CAD build for the part. Positions are in the model's coordinates, mm. A direction names the side the tool comes from. Coordinates: 2 decimals unless noted, no trailing zeros. Loops run counter-clockwise (first coordinate to the right, second up) from the corner with the lowest first, then second, coordinate; pieces in that order, holes last. Notation, with made-up numbers: (71, -8.5) -> (98, -8.5) arc R14 cw to (98, 14.5) -> close; hole circle Ø9 at (-27, -40). An arc over 180 degrees is marked (long way). Write item = value, one per line. Start each with the question number.
(1) Drill centre lines: line 1 (Y direction, x = -2.5, z = 6.5); line 2 (X direction, y = 4.5, z = 7.5); line 3 (X direction, y = 8, z = 2.25). Where is each one in solid material? Low to high. Write a range as from..to.
(2) Tool access for faces 1 (the face through (-8.264, 19.366, 2.075)), 2 (the face through (6.115, 17.736, -1.524)), 3 (the face through (1.237, 24.566, 6.484)): list every direction of +Z, -Z, +X, -X, +Y, -Y with a clear straight run to the whole face (end or side of a thin tool).
(3) Band-saw the part on A-A (y = 3.5). Write the cut outline in (x, z).
(4) Band-saw the part on D-D (y = 6.5). Write the cut outline in (x, z), and give its area (3 significant figures).
(5) Pull direction Z, two halves, no side cores. Call faces 4 (the face through (3, 13, -3.839)), 5 (the face through (6.115, 7.986, -1.524)), 6 (the face through (1.59, 13.31, -0.61)): +Z half, -Z half, draft (parallel to the pull), parting line (faces both ways), or undercut.
(6) Band-saw the part on C-C (z = 2). Count the separate pieces of the cut face and the enclosed holes in it, and give its area (3 significant figures).
(7) Band-saw the part on B-B (x = -3.5). Write the cut outline in (y, z), and give its area (3 significant figures).
(8) Flat gauge pin, fed straight in: P1, Ø2.5, axis at x = 9.94, y = 3.5, coming from the -Z side. Where does the tip first touch, or does it go through?
```python
from build123d import *

# Parameters (mm, degrees)
EXTRUDE_1_DEPTH        = 7
SKETCH_2_R             = 5
EXTRUDE_2_DEPTH        = 15
EXTRUDE_3_DEPTH        = 1.25
PATTERN_LINEAR_1_COUNT = 4
PATTERN_LINEAR_1_PITCH = 3.25
EXTRUDE_5_DEPTH        = 5
SKETCH_8_R             = 1.6
CUT_EXTRUDE_2_DEPTH    = 33.583240961
SKETCH_9_R             = 1.5
CUT_EXTRUDE_3_DEPTH    = 5
SKETCH_10_R            = 3
CUT_EXTRUDE_4_DEPTH    = 32.373048931


with BuildPart() as part:
    # 草图1 → 凸台-拉伸1 (new body)
    with BuildSketch(Plane(origin=(0, 0, 0), x_dir=(1, 0, 0), z_dir=(0, 1, 0))):
        with BuildLine():
            Line((-7.264367816, 3.83908046), (12.735632184, 3.83908046))
            ThreePointArc((12.735632184, 3.83908046), (13.735632184, -2.16091954), (12.735632184, -8.16091954))
            Line((12.735632184, -8.16091954), (-7.264367816, -8.16091954))
            ThreePointArc((-7.264367816, -8.16091954), (-8.264367816, -2.16091954), (-7.264367816, 3.83908046))
        make_face()
    extrude(amount=EXTRUDE_1_DEPTH)

    # 草图2 → 凸台-拉伸2 (add)
    with BuildSketch(Plane(origin=(0, 7, 0), x_dir=(1, 0, 0), z_dir=(0, 1, 0))):
        with Locations(Location((2.735632184, -2.16091954, 0), (0, 0, 270))):
            Circle(SKETCH_2_R)
    extrude(amount=EXTRUDE_2_DEPTH)

    # 草图4 → 凸台-拉伸3 (add)
    with BuildSketch(Plane(origin=(0, 9, 0), x_dir=(1, 0, 0), z_dir=(0, 1, 0))):
        with BuildLine():
            Line((-7.264367816, -8.16091954), (12.735632184, -8.16091954))
            ThreePointArc((12.735632184, -8.16091954), (13.735632184, -2.16091954), (12.735632184, 3.83908046))
            Line((12.735632184, 3.83908046), (-7.264367816, 3.83908046))
            ThreePointArc((-7.264367816, 3.83908046), (-8.264367816, -2.16091954), (-7.264367816, -8.16091954))
        make_face()
    extrude_3 = extrude(amount=EXTRUDE_3_DEPTH)

    # 阵列(线性)1: 凸台-拉伸3 ×4
    with Locations(*[(0, i * PATTERN_LINEAR_1_PITCH, 0) for i in range(1, PATTERN_LINEAR_1_COUNT)]):
        add(extrude_3)

    # 草图6 → 凸台-拉伸5 (add)
    with BuildSketch(Plane(origin=(0, 22, 0), x_dir=(1, 0, 0), z_dir=(0, 1, 0))):
        with BuildLine():
            Line((12.735632184, 3.83908046), (-7.264367816, 3.83908046))
            ThreePointArc((-7.264367816, 3.83908046), (-8.264367816, -2.16091954), (-7.264367816, -8.16091954))
            Line((-7.264367816, -8.16091954), (12.735632184, -8.16091954))
            ThreePointArc((12.735632184, -8.16091954), (13.735632184, -2.16091954), (12.735632184, 3.83908046))
        make_face()
    extrude(amount=EXTRUDE_5_DEPTH)

    # 草图8 → 切除-拉伸2 (cut, through all)
    with BuildSketch(Plane.XY.offset(8.16091954)):
        with Locations((-4.364367816, 3.5)):
            Circle(SKETCH_8_R)
        with Locations((9.935632184, 3.5)):
            Circle(SKETCH_8_R)
    extrude(amount=-CUT_EXTRUDE_2_DEPTH, mode=Mode.SUBTRACT)

    # 草图9 → 切除-拉伸3 (cut)
    with BuildSketch(Plane.XY.offset(8.16091954)):
        with Locations((2.735632184, 24.5)):
            Circle(SKETCH_9_R)
    extrude(amount=-CUT_EXTRUDE_3_DEPTH, mode=Mode.SUBTRACT)

    # 草图10 → 切除-拉伸4 (cut, through all)
    with BuildSketch(Plane.XZ):
        with Locations(Location((2.735995225, 2.16091954, 0), (0, 0, 270))):
            Circle(SKETCH_10_R)
    extrude(amount=-CUT_EXTRUDE_4_DEPTH, mode=Mode.SUBTRACT)


solid = part.part
```
Findings below:
q1.line_1 = 0..7, 9..10.25, 12.25..13.5, 15.5..16.75, 18.75..20, 22..27
q1.line_2 = -7.48..-5.61, -3.12..8.69, 11.18..12.95
q1.line_3 = -2.26..-0.26, 5.73..7.73
q2.face_1 = -X, +Y, -Y
q2.face_2 = none
q2.face_3 = +Z
q3.outline = (-7.26, -3.84) -> (-5.96, -3.84) -> (-5.96, 8.16) -> (-7.26, 8.16) arc R18.5 ccw to start; (-2.76, -3.84) -> (8.34, -3.84) -> (8.34, 8.16) -> (-2.76, 8.16) -> close; (11.54, -3.84) -> (12.74, -3.84) arc R18.5 ccw to (12.74, 8.16) -> (11.54, 8.16) -> close; hole circle Ø6 at (2.74, 2.16)
q4.outline = (-7.26, -3.84) -> (12.74, -3.84) arc R18.5 ccw to (12.74, 8.16) -> (-7.26, 8.16) arc R18.5 ccw to start; hole circle Ø6 at (2.74, 2.16)
q4.area = 228 mm²
q5.face_4 = -Z half
q5.face_5 = parting line
q5.face_6 = undercut
q6.separate_pieces = 2
q6.enclosed_holes = 2
q6.area = 296 mm²
q7.outline = (0, -3.84) -> (2.15, -3.84) -> (2.15, 8.16) -> (0, 8.16) -> close; (4.85, -3.84) -> (7, -3.84) -> (7, 8.16) -> (4.85, 8.16) -> close; (9, -3.84) -> (10.25, -3.84) -> (10.25, 8.16) -> (9, 8.16) -> close; (12.25, -3.84) -> (13.5, -3.84) -> (13.5, 8.16) -> (12.25, 8.16) -> close; (15.5, -3.84) -> (16.75, -3.84) -> (16.75, 8.16) -> (15.5, 8.16) -> close; (18.75, -3.84) -> (20, -3.84) -> (20, 8.16) -> (18.75, 8.16) -> close; (22, -3.84) -> (27, -3.84) -> (27, 8.16) -> (22, 8.16) -> close
q7.area = 172 mm²
q8.P1 = through
